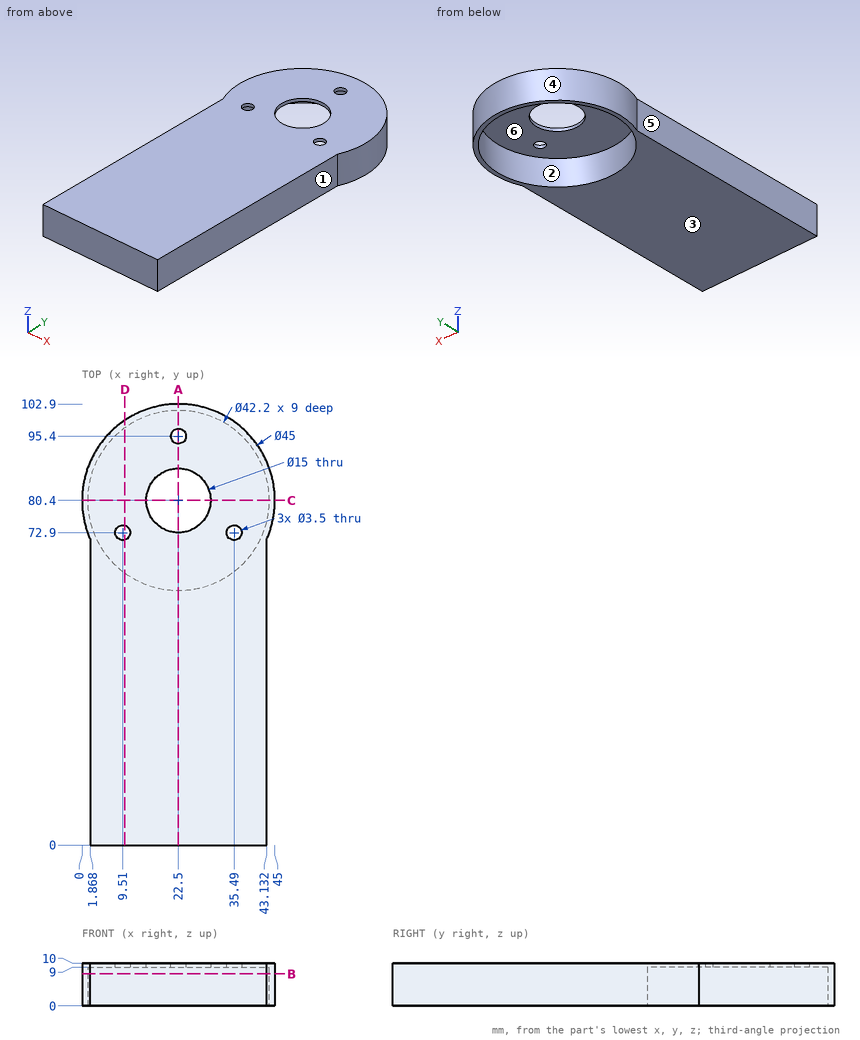
Design review of the part shown in the three views and the two pictorial views. Dimensions are in mm from the part's minimum x, y and z. A direction names the side the tool comes from. Round coordinates to 2 decimals unless told otherwise and drop trailing zeros. Write each loop counter-clockwise with the first axis right and the second up, starting at its lowest first coordinate (ties: lowest second). Pieces come first, ordered by that corner, then holes.
Item 1: For probe 1 along Y at (x, z) = (22.5, 9.65); probe 2 along X at (y, z) = (55.5, 5.25); probe 3 along Y at (x, z) = (22.5, 6), list the stretches that pass through material, from the lowest coordinate up.
Item 2: We need section C-C on y = 80.4. Write out the cut boundary in (x, z).
Item 3: We need section B-B on z = 7.5. Write out the cut boundary in (x, y), and give its area (3 significant figures).
Item 4: The part is to be moulded in two halves that separate along Y. For the marked faces 4, 5 and 6, say which applies: +Y half, -Y half, draft (parallel to the pull), parting line (faces both ways), or undercut.
Item 5: We need section D-D on x = 10. Write out the cut boundary in (y, z).
Item 6: Clearance check with flat-ended pins moving along their axes: pin 1 Ø5.5 at (x, y) = (9.51, 72.9) entering from -Z; pin 2 Ø5 at (y, z) = (33.5, 6) entering from -X; pin 3 Ø6 at (y, z) = (63.5, 5) entering from +X. State where each tip first meets the part, or that it passes through.
Item 7: We need section A-A on x = 22.5. Write out the cut boundary in (y, z), and give its area (3 significant figures).
Item 8: For the marked faces 1, 2 and 3, list the 3-axis set-ups (+Z, -Z, +X, -X, +Y, -Y) from which the entire face can be reached by the end or side of a thin tool; tool diameter is ignored.
Returned:
1. probe 1: y = 0 to 72.9, 87.9 to 93.65, 97.15 to 102.9
1. probe 2: x = 1.87 to 43.13
1. probe 3: y = 0 to 59.3, 101.5 to 102.9
2. outline: (0, 0) - (1.4, 0) - (1.4, 9) - (15, 9) - (15, 10) - (0, 10) - close; (30, 9) - (43.6, 9) - (43.6, 0) - (45, 0) - (45, 10) - (30, 10) - close
3. outline: (1.87, 0) - (43.13, 0) - (43.13, 71.42) arc R22.5 ccw (long way) to (1.87, 71.42) - close; hole circle Ø42.2 at (22.5, 80.4)
3. area: 2,740 mm2
4. face 4: parting line
4. face 5: draft
4. face 6: undercut
5. outline: (0, 0) - (63.4, 0) - (63.4, 9) - (71.22, 9) - (71.22, 10) - (0, 10) - close; (74.58, 9) - (97.4, 9) - (97.4, 0) - (99.11, 0) - (99.11, 10) - (74.58, 10) - close
6. pin 1: stops at z = 9
6. pin 2: stops at x = 1.87
6. pin 3: stops at x = 43.13
7. outline: (0, 0) - (59.3, 0) - (59.3, 9) - (72.9, 9) - (72.9, 10) - (0, 10) - close; (87.9, 9) - (93.65, 9) - (93.65, 10) - (87.9, 10) - close; (97.15, 9) - (101.5, 9) - (101.5, 0) - (102.9, 0) - (102.9, 10) - (97.15, 10) - close
7. area: 631 mm2
8. face 1: +Z, -Z, +X, -Y
8. face 2: -Z
8. face 3: -Z, +X, -X, +Y, -Y
